CAD build for the part. Positions are in the model's coordinates, mm. A direction names the side the tool comes from. Round coordinates to 2 decimals unless told otherwise and drop trailing zeros. Loops run counter-clockwise (first coordinate to the right, second up) from the corner with the lowest first, then second, coordinate; pieces in that order, holes last.
```python
from build123d import *

# Parameters (mm, degrees)
F0_W         = 50
F0_H         = 80
F0_W_2       = 40
F0_H_2       = 70
F1_DEPTH     = 969
F2_W         = 80
F2_H         = 50
F2_W_2       = 70
F2_H_2       = 40
F3_DEPTH     = 914.4
F5_DEPTH     = 50
F6_R         = 17.5
F6_R_2       = 9.5
F7_DEPTH     = 50.001
F8_T         = 5
F8_T3_DEPTH  = 60
F8_T5_DEPTH  = 979
F8_T7_DEPTH  = 924.4
F8_T9_DEPTH  = 80
F8_T11_DEPTH = 50
F9_START     = -25.4
F6_R_3       = 5
F9_DEPTH     = 27.432


# Not quite as in the source:
# - a shell that OpenCascade refuses in one call is made with other operations: the cavity is built on its own and cut out


with BuildPart() as f1:
    # F0 (on Right) → F1 (new body)
    with BuildSketch(Plane.YZ):
        with Locations((-25, 40)):
            Rectangle(F0_W, F0_H)
        with Locations((-25, 40)):
            Rectangle(F0_W_2, F0_H_2, mode=Mode.SUBTRACT)
    extrude(amount=-F1_DEPTH)

    # F2 (on face) → F3 (join)
    with BuildSketch(Plane.XY.offset(80)):
        with Locations((-40, -25)):
            Rectangle(F2_W, F2_H)
        with Locations((-40, -25)):
            Rectangle(F2_W_2, F2_H_2, mode=Mode.SUBTRACT)
    extrude(amount=F3_DEPTH)

    # F4 (on face) → F5 (join)
    with BuildSketch(Plane.XZ.offset(50)):
        Polygon((-80, 994.4), (-969, 80), (-857.4231981277, 80), (-80, 879.6352895028), align=None)
    extrude(amount=-F5_DEPTH)

    # F6 (on face) → F7 (cut, through all)
    with BuildSketch(Plane.XZ.offset(50)):
        with Locations((-581.6838212861, 421)):
            Circle(F6_R)
        with Locations((-913.2115990639, 40)):
            Circle(F6_R_2)
    extrude(amount=-F7_DEPTH, mode=Mode.SUBTRACT)

    # F8: shell of thickness 5, made by hand


with BuildPart() as f8_core1:
    # F8_t2: copy of F1
    add(f1.part)

    # the walls: a layer under each face that stays
    f8_faces = [f8_core1.faces().sort_by_distance(p)[0] for p in [
        (-484.5, -25, 0),
        (-484.5, -50, 497.2),
        (-484.5, 0, 497.2),
        (0, -25, 497.2),
        (-969, -46.4285714286, 5.7142857143),
        (-524.5, -25, 537.2),
        (-74.2857142857, -46.4285714286, 994.4),
        (-922.7115990639, -47.5, 40),
        (-468.7115990639, -25, 80),
        (-80, -25, 479.8176447514),
        (-468.7115990639, -25, 479.8176447514),
        (-922.7115990639, -2.5, 40),
        (-484.5, -25, 75),
        (-484.5, -5, 40),
        (-484.5, -25, 5),
        (-484.5, -45, 40),
        (-40, -5, 537.2),
        (-5, -25, 537.2),
        (-40, -45, 537.2),
        (-75, -25, 537.2),
        (-40, -25, 80),
    ]]
    thicken(f8_faces, amount=-F8_T, mode=Mode.SUBTRACT)

    # F8_s4 → F8_t3 (cut)
    with BuildSketch(Plane.XZ.offset(-5)):
        Polygon((-80.05, 80.05), (-80, 75), (-75, 75), (-75, 80), align=None)
        Polygon((-857.3873483818, 80.0151460803), (-857.4231981277, 75), (-869.2578593558, 75), (-861.0081727218, 83.4853919665), align=None)
        Polygon((-80.0141502541, 879.6004355831), (-75, 879.6352895028), (-75, 891.9509410517), (-83.5849745941, 883.1206814692), align=None)
    extrude(amount=F8_T3_DEPTH, mode=Mode.SUBTRACT)

    # F8_s6 → F8_t5 (cut)
    with BuildSketch(Plane.YZ.offset(-974)):
        Polygon((-44.95, 74.95), (-45, 80), (-50, 80), (-50, 75), align=None)
        Polygon((-5.05, 74.95), (-5, 80), (0, 80), (0, 75), align=None)
        Polygon((-5.05, 5.05), (0, 5), (0, 0), (-5, 0), align=None)
        Polygon((-44.95, 5.05), (-45, 0), (-50, 0), (-50, 5), align=None)
    extrude(amount=F8_T5_DEPTH, mode=Mode.SUBTRACT)

    # F8_s8 → F8_t7 (cut)
    with BuildSketch(Plane.XY.offset(75)):
        Polygon((-74.95, -5.05), (-75, 0), (-80, 0), (-80, -5), align=None)
        Polygon((-5.05, -5.05), (-5, 0), (0, 0), (0, -5), align=None)
        Polygon((-5.05, -44.95), (0, -45), (0, -50), (-5, -50), align=None)
        Polygon((-74.95, -44.95), (-75, -50), (-80, -50), (-80, -45), align=None)
    extrude(amount=F8_T7_DEPTH, mode=Mode.SUBTRACT)

    # F8_s10 → F8_t9 (cut)
    with BuildSketch(Plane.YZ.offset(-80)):
        Polygon((-5.05, 80.05), (0, 80), (0, 75), (-5, 75), align=None)
        Polygon((-44.95, 80.05), (-50, 80), (-50, 75), (-45, 75), align=None)
    extrude(amount=F8_T9_DEPTH, mode=Mode.SUBTRACT)

    # F8_s12 → F8_t11 (cut)
    with BuildSketch(Plane.XZ):
        Polygon((-5.05, 80.05), (0, 80), (0, 75), (-5, 75), align=None)
        Polygon((-74.95, 80.05), (-80, 80), (-80, 75), (-75, 75), align=None)
    extrude(amount=F8_T11_DEPTH, mode=Mode.SUBTRACT)


with BuildPart() as f1_1:
    add(f1.part)

    # what is left inside the walls is the cavity
    f8_cavity = [f8_core1.part.solids().sort_by_distance(p)[0] for p in [
        (-635.349987, -5.05, 363.508502),
    ]]
    add(f8_cavity, mode=Mode.SUBTRACT)

    # F6 (on face) → F9 (cut)
    with BuildSketch(Plane.XZ.offset(50).offset(F9_START)):
        with Locations((-40, 969.4)):
            Circle(F6_R_3)
        with Locations((-40, 944.4)):
            Circle(F6_R_3)
    extrude(amount=-F9_DEPTH, mode=Mode.SUBTRACT)


solid = f1_1.part
```
Item 1: Cut at B-B, the plane z = 421. Give the cut face in (x, y), plus the area to 3 significant figures.
Answers follow:
outline: (-637.47, -50) - (-599.18, -50) - (-599.18, -45) - (-630.5, -45) - (-630.5, -5) - (-599.18, -5) - (-599.18, 0) - (-637.47, 0) - close; (-564.18, -50) - (-525.9, -50) - (-525.9, 0) - (-564.18, 0) - (-564.18, -5) - (-532.87, -5) - (-532.87, -45) - (-564.18, -45) - close; (-80, -50) - (0, -50) - (0, 0) - (-80, 0) - close; hole (-75, -45) - (-5, -45) - (-5, -5) - (-75, -5) - close
area: 2,520 mm2
Item 2: Cut at A-A, the plane y = -25. Give the cut face in (x, z), plus the area to 3 significant figures.
Answers follow:
outline: (-969, 0) - (0, 0) - (0, 5) - (-969, 5) - close; (-969, 75) - (0, 75) - (0, 994.4) - (-5, 994.4) - (-5, 80) - (-75, 80) - (-75, 994.4) - (-80, 994.4) - (-969, 80) - close; hole (-962.03, 80) - (-864.4, 80) - (-80, 886.81) - (-80, 987.23) - close; hole (-857.42, 80) - (-80, 80) - (-80, 879.64) - close
area: 30,800 mm2
Item 3: Two-plate mould, pull along Y, no slides. Class faces 1 (the flat face through (-478, -5, 40)), 2 (the flat face through (0, -25, 490)), 3 (the flat face through (-451, 0, 500)): released by +Y, released by -Y, zero draft, split by the parting line, or undercut.
Answers follow:
face 1: undercut
face 2: zero draft
face 3: released by +Y
Item 4: Probe line 1 (Z direction, x = -40, y = -2.7); line 2 (Z direction, x = -714.5, y = -24.5); line 3 (Z direction, x = -619, y = -35.5). List the from-to ranges inside material, lowest first.
Answers follow:
line 1: z = 0 to 939.4, 949.4 to 964.4, 974.4 to 994.4
line 2: z = 0 to 5, 75 to 80, 227.01 to 234.18, 334.6 to 341.77
line 3: z = 0 to 5, 75 to 80, 325.24 to 332.41, 432.83 to 440
Item 5: Cut at C-C, the plane x = -368.5. Give the cut face in (y, z).
Answers follow:
outline: (-50, 0) - (0, 0) - (0, 80) - (-50, 80) - close; (-50, 582.89) - (0, 582.89) - (0, 697.66) - (-50, 697.66) - close; hole (-45, 5) - (-5, 5) - (-5, 75) - (-45, 75) - close; hole (-45, 590.07) - (-5, 590.07) - (-5, 690.48) - (-45, 690.48) - close
Item 6: 3-axis set-ups, long thin cutter, end or side, ignore diameter. For faces 4 (the flat face through (-478, -25, 5)), 5 (the flat face through (-80, -25, 474)), 6 (the flat face through (-40, -5, 531)): which of +Z, -Z, +X, -X, +Y, -Y reach the whole face in a straight line?
Answers follow:
face 4: +X, -X
face 5: +Y, -Y
face 6: +Z
Item 7: Cut at D-D, the plane z = 811.5. Give the cut face in (x, y), plus the area to 3 significant figures.
Answers follow:
outline: (-257.82, -50) - (-146.24, -50) - (-146.24, 0) - (-257.82, 0) - close; (-80, -50) - (0, -50) - (0, 0) - (-80, 0) - close; hole (-250.85, -45) - (-153.22, -45) - (-153.22, -5) - (-250.85, -5) - close; hole (-75, -45) - (-5, -45) - (-5, -5) - (-75, -5) - close
area: 2,870 mm2
Item 8: Flat gauge pins, fed straight in: P1, Ø21, axis at x = -581.68, z = 421, coming from the -Y side; P2, Ø15, axis at y = -25.5, z = 576, coming from the -X side; P3, Ø3, axis at x = -203, y = -29.5, coming from the +Z side; P4, Ø6, axis at y = -24, z = 434.5, coming from the -X side. Where does each tip first touch, or does it go through?
Answers follow:
P1: passes through
P2: stops at x = -494.07
P3: stops at z = 869.43
P4: stops at x = -627.26
